Geometry: final body of the model. Coordinates: model frame, mm. Face numbers are marked on the shaded views. A direction names the side the tool comes from. Give positions to 0.01 mm unless a question says otherwise; leave off trailing zeros. Write each loop counter-clockwise with the first axis right and the second up, starting at its lowest first coordinate (ties: lowest second). Pieces come first, ordered by that corner, then holes. Notation, with made-up numbers: M 53.25,-29.75 L 66.25,-29.75 A18 ccw 66.25,3.25 Z; hole C -36,79 d6. An arc over 180 degrees is marked long. Use a Markdown table: item, result. Add a question column.
1) Pin query (flat end, axial travel): pin 1 (5 mm diameter, centred on y = 4, z = 5.5, fed in from +X); pin 2 (0.6 mm diameter, centred on x = -2.5, z = -1, fed in from +Y); pin 3 (3 mm diameter, centred on y = 7.5, z = -3.5, fed in from +X). Return the tip coordinate at first contact, or that it passes through.
2) Line query: line 1 (Y direction, x = 2.75, z = -2); line 2 (X direction, y = 1.3, z = 0); line 3 (X direction, y = 10.25, z = 1.25). Output: solid intervals per line, ascending.
3) Section B-B on x = 0. Return the cut outline in (y, z).
4) Set-up query: the marked faces 4 and 5. Return all of +Z, -Z, +X, -X, +Y, -Y with unobstructed straight access to the full face (end or side cutting, diameter ignored); none if empty.
5) Section D-D on y = 19.75. Return the cut outline in (x, z), then the cut area to 3 significant figures.
6) Section A-A on y = 17. Return the cut outline in (x, z).
7) Draft query along X for the marked faces 1, 2 and 3. Return one class per face: +X half, -X half, draft (parallel to the pull), parting line (faces both ways), or undercut.
8) Section C-C on z = 0. Return the cut outline in (x, y).
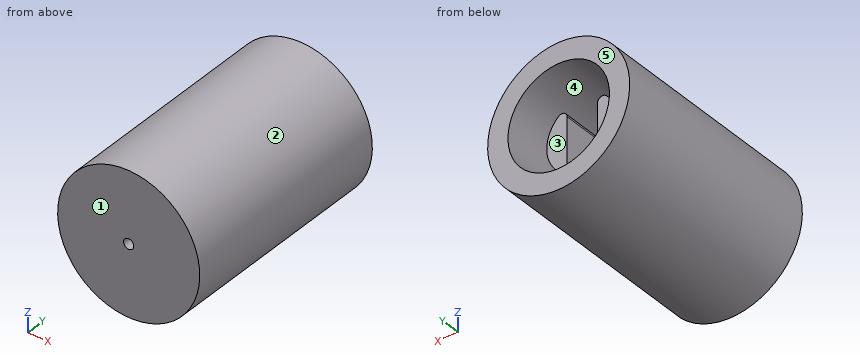
```python
from build123d import *

# Parameters (mm, degrees)
SKETCH1_R           = 7
BOSS_EXTRUDE1_DEPTH = 22
CAVITY1_START       = 2
CAVITY1_OUTLINE_R   = 5
CAVITY1_DEPTH       = 20
CAVITY1_START_2     = 19
CAVITY1_2_DEPTH     = 3
CAVITY1_3_OUTLINE_R = 0.8
CAVITY1_3_DEPTH     = 2
SKETCH2_R           = 0.5
CUT_EXTRUDE1_DEPTH  = 23.315913604


# Read off the part's stored shape, not the designer's step: Cavity1
with BuildPart() as part:
    # Sketch1 → Boss-Extrude1 (new body)
    with BuildSketch(Plane(origin=(0, 0, 0), x_dir=(1, 0, 0), z_dir=(0, 1, 0))):
        with Locations(Location((0, 0, 0), (0, 0, 270))):
            Circle(SKETCH1_R)
    extrude(amount=BOSS_EXTRUDE1_DEPTH)

    # Cavity1 outline → Cavity1 (cut)
    with BuildSketch(Plane(origin=(0, 0, 0), x_dir=(1, 0, 0), z_dir=(0, 1, 0)).offset(CAVITY1_START)):
        Circle(CAVITY1_OUTLINE_R)
        with BuildLine():
            ThreePointArc((-1.5, -2.236067977), (-1.795875854, -2.692503442), (-2.333333333, -2.608745974))
            ThreePointArc((-2.333333333, -2.608745974), (-3.5, 0), (-2.333333333, 2.608745974))
            ThreePointArc((-2.333333333, 2.608745974), (-1.795875854, 2.692503442), (-1.5, 2.236067977))
            Line((-1.5, 2.236067977), (-1.5, -2.236067977))
        make_face(mode=Mode.SUBTRACT)
        with BuildLine():
            Line((1.5, -2.236067977), (1.5, 2.236067977))
            ThreePointArc((1.5, 2.236067977), (1.795875854, 2.692503442), (2.333333333, 2.608745974))
            ThreePointArc((2.333333333, 2.608745974), (3.5, 0), (2.333333333, -2.608745974))
            ThreePointArc((2.333333333, -2.608745974), (1.795875854, -2.692503442), (1.5, -2.236067977))
        make_face(mode=Mode.SUBTRACT)
    extrude(amount=CAVITY1_DEPTH, mode=Mode.SUBTRACT)

    # Cavity1 2 outline → Cavity1 2 (cut)
    with BuildSketch(Plane(origin=(0, 0, 0), x_dir=(1, 0, 0), z_dir=(0, 1, 0)).offset(CAVITY1_START_2)):
        with BuildLine():
            ThreePointArc((2.333333333, 2.608745974), (1.795875854, 2.692503442), (1.5, 2.236067977))
            Line((1.5, 2.236067977), (1.5, -2.236067977))
            ThreePointArc((1.5, -2.236067977), (1.795875854, -2.692503442), (2.333333333, -2.608745974))
            ThreePointArc((2.333333333, -2.608745974), (3.5, 0), (2.333333333, 2.608745974))
        make_face()
        with BuildLine():
            ThreePointArc((-2.333333333, 2.608745974), (-3.5, 0), (-2.333333333, -2.608745974))
            ThreePointArc((-2.333333333, -2.608745974), (-1.795875854, -2.692503442), (-1.5, -2.236067977))
            Line((-1.5, -2.236067977), (-1.5, 2.236067977))
            ThreePointArc((-1.5, 2.236067977), (-1.795875854, 2.692503442), (-2.333333333, 2.608745974))
        make_face()
    extrude(amount=CAVITY1_2_DEPTH, mode=Mode.SUBTRACT)

    # Cavity1 3 outline → Cavity1 3 (cut)
    # profile 1 of 2: a face of its own
    with BuildSketch(Plane(origin=(0, 0, 0), x_dir=(1, 0, 0), z_dir=(0, 1, 0)).offset(CAVITY1_START)):
        with BuildLine():
            ThreePointArc((2.333333333, 2.608745974), (1.795875854, 2.692503442), (1.5, 2.236067977))
            Line((1.5, 2.236067977), (1.5, -2.236067977))
            ThreePointArc((1.5, -2.236067977), (1.795875854, -2.692503442), (2.333333333, -2.608745974))
            ThreePointArc((2.333333333, -2.608745974), (3.5, 0), (2.333333333, 2.608745974))
        make_face()
        with Locations((2.5, 0)):
            Circle(CAVITY1_3_OUTLINE_R, mode=Mode.SUBTRACT)
    # profile 2 of 2: a face of its own
    with BuildSketch(Plane(origin=(0, 0, 0), x_dir=(1, 0, 0), z_dir=(0, 1, 0)).offset(CAVITY1_START)):
        with BuildLine():
            ThreePointArc((-2.333333333, 2.608745974), (-3.5, 0), (-2.333333333, -2.608745974))
            ThreePointArc((-2.333333333, -2.608745974), (-1.795875854, -2.692503442), (-1.5, -2.236067977))
            Line((-1.5, -2.236067977), (-1.5, 2.236067977))
            ThreePointArc((-1.5, 2.236067977), (-1.795875854, 2.692503442), (-2.333333333, 2.608745974))
        make_face()
        with Locations((-2.5, 0)):
            Circle(CAVITY1_3_OUTLINE_R, mode=Mode.SUBTRACT)
    extrude(amount=CAVITY1_3_DEPTH, mode=Mode.SUBTRACT)

    # Sketch2 → Cut-Extrude1 (cut, through all)
    with BuildSketch(Plane(origin=(0, 2, 0), x_dir=(1, 0, 0), z_dir=(0, 1, 0))):
        with Locations(Location((0, 0, 0), (0, 0, 270))):
            Circle(SKETCH2_R)
    extrude(amount=-CUT_EXTRUDE1_DEPTH, mode=Mode.SUBTRACT)


solid = part.part
```
Found:
| question | item | result |
|---|---|---|
| 1 | pin 1 | x = 6.32 |
| 1 | pin 2 | y = 19 |
| 1 | pin 3 | x = 6.71 |
| 2 | line 1 | 0 to 2, 4 to 19 |
| 2 | line 2 | -7 to -0.5, 0.5 to 7 |
| 2 | line 3 | -6.89 to -4.84, -3.27 to -1.5, 1.5 to 3.27, 4.84 to 6.89 |
| 3 | outline | M 0,-7 L 22,-7 L 22,-5 L 2,-5 L 2,-0.5 L 0,-0.5 Z; M 0,0.5 L 2,0.5 L 2,5 L 22,5 L 22,7 L 0,7 Z |
| 4 | face 4 | +Y |
| 4 | face 5 | +Z, -Z, +X, -X, +Y |
| 5 | outline | C 0,0 d14; hole C 0,0 d10 |
| 5 | area | 75.4 mm² |
| 6 | outline | C 0,0 d14; M -2.33,-2.61 A0.5 ccw -1.5,-2.24 L -1.5,2.24 A0.5 ccw -2.33,2.61 A3.5 ccw Z; M 1.5,-2.24 A0.5 ccw 2.33,-2.61 A3.5 ccw 2.33,2.61 A0.5 ccw 1.5,2.24 Z; hole C 0,0 d10 |
| 7 | face 1 | draft |
| 7 | face 2 | parting line |
| 7 | face 3 | undercut |
| 8 | outline | M -7,0 L -0.5,0 L -0.5,2 L -1.7,2 L -1.7,4 L -1.5,4 L -1.5,19 L -3.5,19 L -3.5,4 L -3.3,4 L -3.3,2 L -5,2 L -5,22 L -7,22 Z; M 0.5,0 L 7,0 L 7,22 L 5,22 L 5,2 L 3.3,2 L 3.3,4 L 3.5,4 L 3.5,19 L 1.5,19 L 1.5,4 L 1.7,4 L 1.7,2 L 0.5,2 Z |
